The figure shows three views and two pictorial views of one solid part (mm, origin at its lowest corner). Answer the questions. A direction names the side the tool comes from. Coordinates: 2 decimals unless noted, no trailing zeros. Order: outer loops, then holes, each group sorted by start corner. A loop starts at its lowest first (then second) coordinate and runs counter-clockwise, first axis right, second up. Notation, with made-up numbers: (64, 59) -> (80, 59) arc R7 ccw to (80, 72) -> close; hole circle Ø5 at (-27.5, -4.5). An arc over 180 degrees is marked (long way). Return JSON: item names as keys, results as strings. Group by question number.
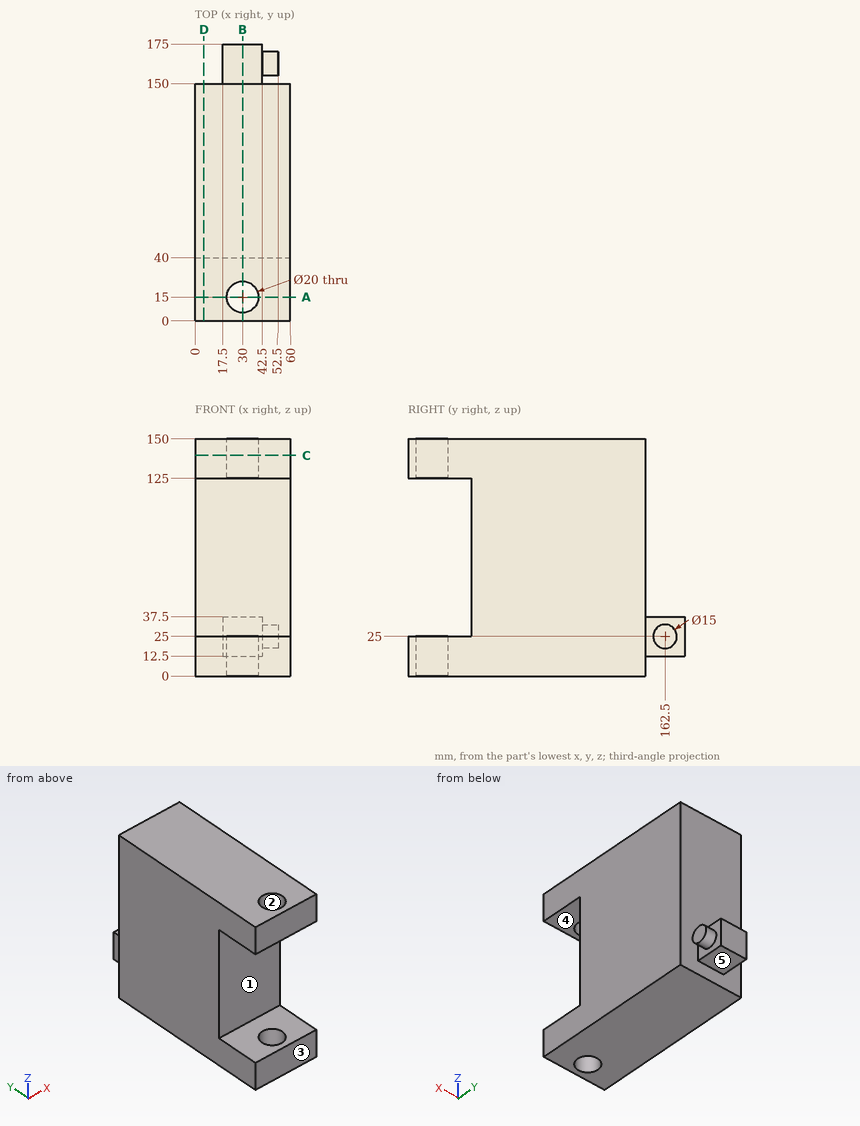
1. Find section A-A on y = 15. Determine the outline of the cut face in (x, z), and give its area (3 significant figures).
2. Find section D-D on x = 5.5. Determine the outline of the cut face in (y, z), and give its area (3 significant figures).
3. Find section B-B on x = 30. Determine the outline of the cut face in (y, z).
4. Given pin 1 (4.5 mm diameter, centred on y = 160.5, z = 28.5, fed in from +X); pin 2 (1 mm diameter, centred on x = 41.5, z = 87, fed in from -Y); pin 3 (5 mm diameter, centred on x = 8, z = 60.5, fed in from +Y), each flat-ended and moving along its own axis, determine where each tip first touches the part or whether it passes through.
5. For a pull along Z with two mould halves and no side action, classify the marked faces 3, 4 and 5 as released by +Z, released by -Z, zero draft, split by the parting line, or undercut.
6. Straight lines are drawn through the part: L1, parallel to Y at x = 30, z = 131; L2, parallel to Z at x = 25, y = 150.5; L3, parallel to Y at x = 18, z = 11. For each, find the intervals that lie inside material, in ascending order.
7. Find section C-C on z = 139.5. Determine the outline of the cut face in (x, y).
8. Which of the six approach directions +Z, -Z, +X, -X, +Y, -Y give full straight-line access (tool end or side, diameter ignored) to the marked faces 1 and 2?
Result:
{
 "1": {"outline": "(0, 0) -> (20, 0) -> (20, 25) -> (0, 25) -> close; (0, 125) -> (20, 125) -> (20, 150) -> (0, 150) -> close; (40, 0) -> (60, 0) -> (60, 25) -> (40, 25) -> close; (40, 125) -> (60, 125) -> (60, 150) -> (40, 150) -> close", "area": "2,000 mm^2"},
 "2": {"outline": "(0, 0) -> (150, 0) -> (150, 150) -> (0, 150) -> (0, 125) -> (40, 125) -> (40, 25) -> (0, 25) -> close", "area": "18,500 mm^2"},
 "3": {"outline": "(0, 0) -> (5, 0) -> (5, 25) -> (0, 25) -> close; (0, 125) -> (5, 125) -> (5, 150) -> (0, 150) -> close; (25, 0) -> (150, 0) -> (150, 12.5) -> (175, 12.5) -> (175, 37.5) -> (150, 37.5) -> (150, 150) -> (25, 150) -> (25, 125) -> (40, 125) -> (40, 25) -> (25, 25) -> close"},
 "4": {"pin 1": "x = 52.5", "pin 2": "y = 40", "pin 3": "y = 150"},
 "5": {"face 3": "zero draft", "face 4": "undercut", "face 5": "released by -Z"},
 "6": {"L1": "0 to 5, 25 to 150", "L2": "12.5 to 37.5", "L3": "0 to 150"},
 "7": {"outline": "(0, 0) -> (60, 0) -> (60, 150) -> (0, 150) -> close; hole circle Ø20 at (30, 15)"},
 "8": {"face 1": "+X, -X, -Y", "face 2": "+Z, -Z"}
}
